from build123d import *

# Parameters (mm, degrees)
CYLINDER101_R     = 1.6
CYLINDER101_DEPTH = 3
CYLINDER102_R     = 1.6
CYLINDER102_DEPTH = 3
CYLINDER103_R     = 1.6
CYLINDER103_DEPTH = 3
CYLINDER145_R     = 1.6
CYLINDER145_DEPTH = 3
CYLINDER146_R     = 1.6
CYLINDER146_DEPTH = 3
CYLINDER100_R     = 1.6
CYLINDER100_DEPTH = 3
BOX079_W          = 32
BOX079_H          = 7
BOX079_DEPTH      = 2
BOX014_W          = 32
BOX014_H          = 40
BOX014_DEPTH      = 2
BOX080_W          = 32
BOX080_H          = 7
BOX080_DEPTH      = 2
BOX078_W          = 32
BOX078_H          = 15
BOX078_DEPTH      = 2
CYLINDER_R        = 4
CYLINDER_DEPTH    = 10
BOX077_W          = 32
BOX077_H          = 15
BOX077_DEPTH      = 2
CHAMFER003_SIZE   = 1


with BuildPart() as cylinder101:
    # Cylinder101 → Cylinder101 (new body)
    with BuildSketch(Plane(origin=(47.5, -22, 7), x_dir=(1, 0, 0), z_dir=(0, 0, 1))):
        Circle(CYLINDER101_R)
    extrude(amount=CYLINDER101_DEPTH)


with BuildPart() as cylinder102:
    # Cylinder102 → Cylinder102 (new body)
    with BuildSketch(Plane(origin=(47.5, -68, 7), x_dir=(1, 0, 0), z_dir=(0, 0, 1))):
        Circle(CYLINDER102_R)
    extrude(amount=CYLINDER102_DEPTH)


with BuildPart() as cylinder103:
    # Cylinder103 → Cylinder103 (new body)
    with BuildSketch(Plane(origin=(27.5, -68, 7), x_dir=(1, 0, 0), z_dir=(0, 0, 1))):
        Circle(CYLINDER103_R)
    extrude(amount=CYLINDER103_DEPTH)


with BuildPart() as cylinder145:
    # Cylinder145 → Cylinder145 (new body)
    with BuildSketch(Plane(origin=(27, -37, 15), x_dir=(1, 0, 0), z_dir=(0, 0, 1))):
        Circle(CYLINDER145_R)
    extrude(amount=CYLINDER145_DEPTH)


with BuildPart() as cylinder146:
    # Cylinder146 → Cylinder146 (new body)
    with BuildSketch(Plane(origin=(27, -53.25, 15), x_dir=(1, 0, 0), z_dir=(0, 0, 1))):
        Circle(CYLINDER146_R)
    extrude(amount=CYLINDER146_DEPTH)


with BuildPart() as fusion046:
    # Cylinder100 → Cylinder100 (new body)
    with BuildSketch(Plane(origin=(27.5, -22, 7), x_dir=(1, 0, 0), z_dir=(0, 0, 1))):
        Circle(CYLINDER100_R)
    extrude(amount=CYLINDER100_DEPTH)

    # Fusion046: union Cylinder101, Cylinder102, Cylinder103, Cylinder145, Cylinder146
    add(cylinder101.part)
    add(cylinder102.part)
    add(cylinder103.part)
    add(cylinder145.part)
    add(cylinder146.part)


with BuildPart() as fusion046_1:
    # Fusion046 placement: moved
    add(fusion046.part.moved(Location((0, 25, 9))))


with BuildPart() as cube079:
    # Box079 → Box079 (new body)
    with BuildSketch(Plane(origin=(21.5, 0, 18), x_dir=(1, 0, 0), z_dir=(0, -1, 0))):
        with Locations((16, 3.5)):
            Rectangle(BOX079_W, BOX079_H)
    extrude(amount=BOX079_DEPTH)


with BuildPart() as cube014:
    # Box014 → Box014 (new body)
    with BuildSketch(Plane(origin=(21.5, -40, 25), x_dir=(1, 0, 0), z_dir=(0, 0, 1))):
        with Locations((16, 20)):
            Rectangle(BOX014_W, BOX014_H)
    extrude(amount=BOX014_DEPTH)


with BuildPart() as cube080:
    # Box080 → Box080 (new body)
    with BuildSketch(Plane(origin=(21.5, -38, 18), x_dir=(1, 0, 0), z_dir=(0, -1, 0))):
        with Locations((16, 3.5)):
            Rectangle(BOX080_W, BOX080_H)
    extrude(amount=BOX080_DEPTH)


with BuildPart() as cube078:
    # Box078 → Box078 (new body)
    with BuildSketch(Plane(origin=(21.5, -53, 16), x_dir=(1, 0, 0), z_dir=(0, 0, 1))):
        with Locations((16, 7.5)):
            Rectangle(BOX078_W, BOX078_H)
    extrude(amount=BOX078_DEPTH)


with BuildPart() as cylinder:
    # Cylinder → Cylinder (new body)
    with BuildSketch(Plane(origin=(37, -20, 27), x_dir=(1, 0, 0), z_dir=(0, 0, 1))):
        Circle(CYLINDER_R)
    extrude(amount=CYLINDER_DEPTH)


with BuildPart() as chamfer003:
    # Box077 → Box077 (new body)
    with BuildSketch(Plane(origin=(21.5, -2, 16), x_dir=(1, 0, 0), z_dir=(0, 0, 1))):
        with Locations((16, 7.5)):
            Rectangle(BOX077_W, BOX077_H)
    extrude(amount=BOX077_DEPTH)

    # Fusion105: union Cube079, Cube014, Cube080, Cube078, Cylinder
    add(cube079.part)
    add(cube014.part)
    add(cube080.part)
    add(cube078.part)
    add(cylinder.part)

    # Cut083: cut Fusion046
    add(fusion046_1.part, mode=Mode.SUBTRACT)

    # Chamfer003
    chamfer003_edges = [chamfer003.edges().sort_by_distance(p)[0] for p in [
        (37.5, -2, 25),
        (37.5, -38, 25),
    ]]
    chamfer(chamfer003_edges, length=CHAMFER003_SIZE)


solid = chamfer003.part
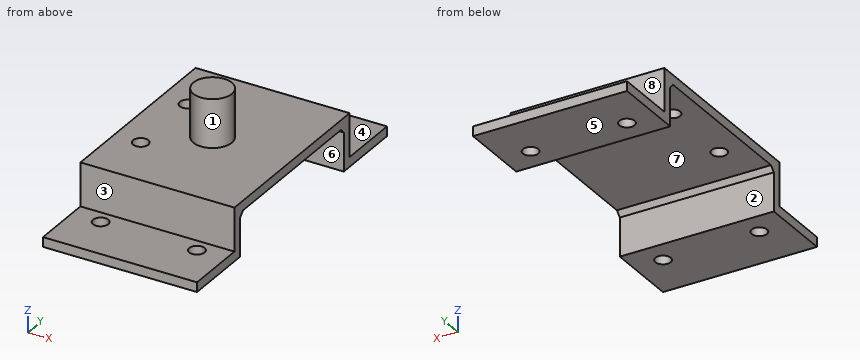
Source: CAD feature listing. Evaluate the final solid. Frame: model axes, mm. Face numbers are marked on the shaded views. A direction names the side the tool comes from. Give positions to 0.01 mm unless a question says otherwise; leave off trailing zeros. Write each loop counter-clockwise with the first axis right and the second up, starting at its lowest first coordinate (ties: lowest second). Pieces come first, ordered by that corner, then holes. Notation, with made-up numbers: (2.25, 30.25) -> (38.25, 30.25) arc R17 ccw to (38.25, 42.25) -> close; hole circle Ø11 at (52.25, 80). An arc over 180 degrees is marked (long way). Return JSON: item names as keys, results as strings. Group by question number.
1. Material intervals for line 1 (X direction, y = 3, z = 17); line 2 (Y direction, x = 47.5, z = 16.8); line 3 (X direction, y = -28.25, z = 25.4), sorted ascending. Write a range as from..to.
2. Section D-D, the plane y = -43. Output: boundary loops of the cut face in (x, z).
3. Mould query, pull axis Y, two halves, no side actions, for the marked faces 5, 6, 7 and 8. Classes: +Y half, -Y half, draft (parallel to the pull), parting line (faces both ways), or undercut.
4. Access query for the marked faces 1, 2, 3 and 4. Directions: +Z, -Z, +X, -X, +Y, -Y. A direction counts if a zero-diameter tool reaches every point of the face in a straight line with its end or side. Return the directions, or none.
5. Section B-B, the plane y = -12. Output: boundary loops of the cut face in (x, z), then the cut area to 3 significant figures.
6. Section A-A, the plane z = 18.75. Output: boundary loops of the cut face in (x, y).
7. Pin query (flat end, axial travel): pin 1 Ø1 at (x, z) = (35, 26.5) entering from -Y; pin 2 Ø6 at (x, y) = (37.5, -23.5) entering from -Z; pin 3 Ø8 at (y, z) = (-28, 22) entering from +X; pin 4 Ø7 at (x, z) = (42.5, 22.5) entering from +Y. Return the tip coordinate at first contact, or that it passes through.
8. Section C-C, the plane x = 47.5. Output: boundary loops of the cut face in (y, z).
Determined:
{
 "1": {"line 1": "x = 21.5..25.9, 29.1..45.9, 49.1..53.5", "line 2": "y = -53..-44.6, -41.4..-38, -2..1.4, 4.6..13", "line 3": "x = 21.5..25.4, 28.6..53.5"},
 "2": {"outline": "(21.5, 16) -> (25.9, 16) -> (25.9, 18) -> (21.5, 18) -> close; (29.1, 16) -> (45.9, 16) -> (45.9, 18) -> (29.1, 18) -> close; (49.1, 16) -> (53.5, 16) -> (53.5, 18) -> (49.1, 18) -> close"},
 "3": {"face 5": "draft", "face 6": "undercut", "face 7": "undercut", "face 8": "+Y half"},
 "4": {"face 1": "+Z", "face 2": "-Z, +X, -X", "face 3": "+Z, +X, -X, -Y", "face 4": "+Z, +X, -X, +Y"},
 "5": {"outline": "(21.5, 25) -> (25.4, 25) -> (25.4, 27) -> (21.5, 27) -> close; (28.6, 25) -> (53.5, 25) -> (53.5, 27) -> (28.6, 27) -> close", "area": "57.6 mm2"},
 "6": {"outline": "(21.5, -40) -> (53.5, -40) -> (53.5, -38) -> (21.5, -38) -> close; (21.5, -2) -> (53.5, -2) -> (53.5, 0) -> (21.5, 0) -> close"},
 "7": {"pin 1": "stops at y = -40", "pin 2": "stops at z = 25", "pin 3": "stops at x = 53.5", "pin 4": "stops at y = 0"},
 "8": {"outline": "(-53, 16) -> (-44.6, 16) -> (-44.6, 18) -> (-53, 18) -> close; (-41.4, 16) -> (-38, 16) -> (-38, 24) -> (-37, 25) -> (-3, 25) -> (-2, 24) -> (-2, 16) -> (1.4, 16) -> (1.4, 18) -> (0, 18) -> (0, 27) -> (-40, 27) -> (-40, 18) -> (-41.4, 18) -> close; (4.6, 16) -> (13, 16) -> (13, 18) -> (4.6, 18) -> close"}
}
